The listing builds one solid part. Answer for the finished solid, in the listing's coordinates (mm). Face numbers are marked on the shaded views. A direction names the side the tool comes from. Round coordinates to 2 decimals unless told otherwise and drop trailing zeros. Loops run counter-clockwise (first coordinate to the right, second up) from the corner with the lowest first, then second, coordinate; pieces in that order, holes last. Notation, with made-up numbers: M -29,14 L -7,14 A12 ccw -7,27 Z; hole C -8,17.25 d5. An arc over 180 degrees is marked long. Answer as a JSON object with one key per item and string values.
```python
from build123d import *

# Parameters (mm, degrees)
M3_CLEARANCE_HOLE1_D   = 3.4
CIRPATTERN1_COUNT      = 4
BOSS_EXTRUDE1_START    = -8.82278
BOSS_EXTRUDE1_DEPTH    = 8.82278
CHAMFER1_SIZE          = 0.75
CHAMFER2_SIZE          = 1
MOVE_START             = 8.11328
MOVE_FACE1_OUTLINE_R   = 8.9
MOVE_FACE1_OUTLINE_R_2 = 8.75
MOVE_FACE1_DEPTH       = 3.223364194


# Read off the part's stored shape, not the designer's step: Move Face1
with BuildPart() as part:
    # Sketch1 → Revolve1 (revolve)
    with BuildSketch(Plane.XY, mode=Mode.PRIVATE) as revolve1_sk:
        Polygon((6.8, 0), (6.8, 4.953), (5.2, 4.953), (5.2, 13.77578), (7.112, 13.77578), (8.9, 11.11328), (8.9, 8.11328), (23, 8.11328), (23, 0), align=None)
    revolve(revolve1_sk.sketch.rotate(Axis((0, 0, 0), (0, 1, 0)), 90), axis=Axis((0, 0, 0), (0, 1, 0)))

    # M3 Clearance Hole1 (through all)
    with Locations(Plane.XZ):
        with Locations((-20, 0)):
            m3_clearance_hole1 = Hole(M3_CLEARANCE_HOLE1_D / 2)

    # CirPattern1: M3 Clearance Hole1 ×4 about axis
    cirpattern1_axis = Axis((0, 0, 0), (0, 1, 0))
    for i in range(1, CIRPATTERN1_COUNT):
        add(m3_clearance_hole1.rotate(cirpattern1_axis, i * 360 / CIRPATTERN1_COUNT), mode=Mode.SUBTRACT)

    # Sketch4 → Boss-Extrude1 (add)
    with BuildSketch(Plane.XZ.offset(-4.953).offset(BOSS_EXTRUDE1_START)):
        with BuildLine():
            Line((0.700412138, 5.152613205), (4.112087862, 3.182881307))
            ThreePointArc((4.112087862, 3.182881307), (2.6, 4.5033321), (0.700412138, 5.152613205))
        make_face()
        with BuildLine():
            ThreePointArc((4.8125, -1.969731898), (5.2, 0), (4.8125, 1.969731898))
            Line((4.8125, 1.969731898), (4.8125, -1.969731898))
        make_face()
        with BuildLine():
            Line((-4.112087862, 3.182881307), (-0.700412138, 5.152613205))
            ThreePointArc((-0.700412138, 5.152613205), (-2.6, 4.5033321), (-4.112087862, 3.182881307))
        make_face()
        with BuildLine():
            ThreePointArc((0.700412138, -5.152613205), (2.6, -4.5033321), (4.112087862, -3.182881307))
            Line((4.112087862, -3.182881307), (0.700412138, -5.152613205))
        make_face()
        with BuildLine():
            Line((-4.8125, -1.969731898), (-4.8125, 1.969731898))
            ThreePointArc((-4.8125, 1.969731898), (-5.2, 0), (-4.8125, -1.969731898))
        make_face()
        with BuildLine():
            ThreePointArc((-4.112087862, -3.182881307), (-2.6, -4.5033321), (-0.700412138, -5.152613205))
            Line((-0.700412138, -5.152613205), (-4.112087862, -3.182881307))
        make_face()
    extrude(amount=BOSS_EXTRUDE1_DEPTH)

    # Chamfer1
    chamfer1_edges = [part.edges().sort_by_distance(p)[0] for p in [
        (0, 0, 6.8),
    ]]
    chamfer(chamfer1_edges, length=CHAMFER1_SIZE)

    # Chamfer2
    chamfer2_edges = [part.edges().sort_by_distance(p)[0] for p in [
        (0, 8.11328, 23),
    ]]
    chamfer(chamfer2_edges, length=CHAMFER2_SIZE)

    # Move Face1 outline → Move Face1 (cut)
    with BuildSketch(Plane(origin=(0, 0, 0), x_dir=(1, 0, 0), z_dir=(0, 1, 0)).offset(MOVE_START)):
        Circle(MOVE_FACE1_OUTLINE_R)
        Circle(MOVE_FACE1_OUTLINE_R_2, mode=Mode.SUBTRACT)
    extrude(amount=MOVE_FACE1_DEPTH, mode=Mode.SUBTRACT)


solid = part.part
```
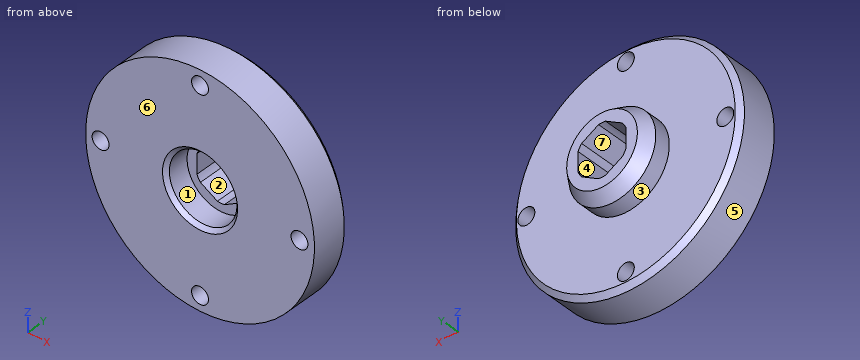
Item 1: The part is cut by section D-D (y = 9.75). Give the vertices of the cut face in (x, z), then the cut area to 3 significant figures.
Values follow:
{"outline": "C 0,0 d17.5; hole M -4.81,-1.97 A5.2 ccw -4.11,-3.18 L -0.7,-5.15 A5.2 ccw 0.7,-5.15 L 4.11,-3.18 A5.2 ccw 4.81,-1.97 L 4.81,1.97 A5.2 ccw 4.11,3.18 L 0.7,5.15 A5.2 ccw -0.7,5.15 L -4.11,3.18 A5.2 ccw -4.81,1.97 Z", "area": "162 mm^2"}
Item 2: Determine the mould class of the marked faces 4, 5, 6 and 7 for opening direction X: released by +X, released by -X, zero draft, split by the parting line, or undercut.
Values follow:
{"face 4": "undercut", "face 5": "split by the parting line", "face 6": "zero draft", "face 7": "undercut"}
Item 3: Which of the six approach directions +Z, -Z, +X, -X, +Y, -Y give full straight-line access (tool end or side, diameter ignored) to the marked faces 1, 2 and 3?
Values follow:
{"face 1": "-Y", "face 2": "+Y, -Y", "face 3": "+Y"}
Item 4: The part is cut by section A-A (z = 0). Give the number of separate pieces and of enclosed holes in the cut face, then the cut area to 3 significant figures.
Values follow:
{"separate pieces": "4", "enclosed holes": "0", "area": "259 mm^2"}
Item 5: Straight lines are drawn through the part: line 1 (Y direction, x = -13.5, z = 5); line 2 (X direction, y = 2.75, z = 3.5); line 3 (Z direction, x = 20, y = 4.5). For each, find the intervals that lie inside material, in ascending order.
Values follow:
{"line 1": "0 to 8.11", "line 2": "-22.73 to -5.83, 5.83 to 22.73", "line 3": "-11.36 to -1.7, 1.7 to 11.36"}
Item 6: Flat-ended cylindrical pins translate along their axes: P1, Ø6, axis at x = -16, z = 14.5, coming from the +Y side; P2, Ø3, axis at x = -11.5, y = 8, coming from the +Z side; P3, Ø1.2, axis at y = 9.5, z = -0.5, coming from the +X side; P4, Ø3, axis at x = -13, z = 10, coming from the -Y side. Find the tip coordinate at first contact, or state that the pin passes through.
Values follow:
{"P1": "y = 8.11", "P2": "z = 20.57", "P3": "x = 8.75", "P4": "y = 0"}
Item 7: The part is cut by section C-C (y = 6.25). Give the vertices of the cut face in (x, z), then the cut area to 3 significant figures.
Values follow:
{"outline": "C 0,0 d46; hole C -20,0 d3.4; hole M -4.81,-1.97 A5.2 ccw -4.11,-3.18 L -0.7,-5.15 A5.2 ccw 0.7,-5.15 L 4.11,-3.18 A5.2 ccw 4.81,-1.97 L 4.81,1.97 A5.2 ccw 4.11,3.18 L 0.7,5.15 A5.2 ccw -0.7,5.15 L -4.11,3.18 A5.2 ccw -4.81,1.97 Z; hole C 0,-20 d3.4; hole C 0,20 d3.4; hole C 20,0 d3.4", "area": "1,550 mm^2"}
